from build123d import *

# Parameters (mm, degrees)
SKETCH1_W                                         = 211
SKETCH1_H                                         = 36
BOSS_EXTRUDE1_DEPTH                               = 18
CUT_EXTRUDE1_DEPTH                                = 4
LPATTERN1_COUNT                                   = 9
LPATTERN1_PITCH                                   = 24.4
CBORE_FOR_M2_5_SOCKET_HEAD_CAP_SCREW1_D           = 2.9
CBORE_FOR_M2_5_SOCKET_HEAD_CAP_SCREW1_CBORE_D     = 5.5
CBORE_FOR_M2_5_SOCKET_HEAD_CAP_SCREW1_CBORE_DEPTH = 2.9
FILLET1_R                                         = 2


with BuildPart() as part:
    # Sketch1 → Boss-Extrude1 (new body)
    with BuildSketch(Plane(origin=(0, 0, 0), x_dir=(1, 0, 0), z_dir=(0, 1, 0))):
        Rectangle(SKETCH1_W, SKETCH1_H)
    extrude(amount=BOSS_EXTRUDE1_DEPTH)

    # Sketch2 → Cut-Extrude1 (cut)
    with BuildSketch(Plane(origin=(0, 18, 0), x_dir=(1, 0, 0), z_dir=(0, 1, 0))):
        with BuildLine():
            Line((-101.6, 9.25), (-101.6, -9.25))
            ThreePointArc((-101.6, -9.25), (-97.6, -13.25), (-93.6, -9.25))
            Line((-93.6, -9.25), (-93.6, 9.25))
            ThreePointArc((-93.6, 9.25), (-97.6, 13.25), (-101.6, 9.25))
        make_face()
    cut_extrude1 = extrude(amount=-CUT_EXTRUDE1_DEPTH, mode=Mode.SUBTRACT)

    # LPattern1: Cut-Extrude1 ×9
    with Locations(*[(i * LPATTERN1_PITCH, 0, 0) for i in range(1, LPATTERN1_COUNT)]):
        add(cut_extrude1, mode=Mode.SUBTRACT)

    # CBORE for M2.5 Socket Head Cap Screw1 (through all)
    with Locations(Plane(origin=(0, 18, 0), x_dir=(1, 0, 0), z_dir=(0, 1, 0))):
        with Locations((-85.4, 0), (85.4, 0)):
            CounterBoreHole(CBORE_FOR_M2_5_SOCKET_HEAD_CAP_SCREW1_D / 2, CBORE_FOR_M2_5_SOCKET_HEAD_CAP_SCREW1_CBORE_D / 2, CBORE_FOR_M2_5_SOCKET_HEAD_CAP_SCREW1_CBORE_DEPTH)

    # Fillet1
    fillet1_edges = [part.edges().sort_by_distance(p)[0] for p in [
        (105.5, 9, 18),
        (-105.5, 9, 18),
        (-105.5, 9, -18),
        (105.5, 9, -18),
    ]]
    fillet(fillet1_edges, radius=FILLET1_R)


solid = part.part
The model under review builds one solid part; all positions refer to its coordinate system, in mm. A direction names the side the tool comes from. Give positions to 0.01 mm unless a question says otherwise; leave off trailing zeros. Order: outer loops, then holes, each group sorted by start corner. A loop starts at its lowest first (then second) coordinate and runs counter-clockwise, first axis right, second up. Notation, with made-up numbers: M -39,9 L 7,9 A30 ccw 7,45 Z; hole C -33.75,48.5 d6. An arc over 180 degrees is marked long. Use one line per item in the form item = value. Start each with the question number.
Item 1: For faces 1 (the flat face through (-1, 9, 18)), 2 (the flat face through (-49, 14, 0)), list the 3-axis set-ups (+Z, -Z, +X, -X, +Y, -Y) from which the entire face can be reached by the end or side of a thin tool; tool diameter is ignored.
Item 2: We need section A-A on x = -73.2. Give the boundary of the cut face in (y, z).
Item 3: Insertion check: pin 1 Ø2.5 at (x, z) = (-25, -6) entering from +Y; pin 2 Ø3 at (x, z) = (86, -1) entering from +Y. Each pin has a flat end and moves straight along its axis. Give the tip position at first contact, or say it passes through.
Item 4: The part is to be moulded in two halves that separate along X. For faces 3 (the cylindrical face through (97.69, 16.03, -13.25)), 4 (the flat face through (105.5, 9, 0)), 5 (the flat face through (-1, 0, 0)), 6 (the flat face through (98, 14, 0)), say which applies: pulls with the +X half, pulls with the -X half, needs draft (parallel to the pull), parting line crosses it, or undercut.
Item 5: To check wall thickness, follow line 1 along Z through (x, y) = (-85.4, 12.25); line 2 along Z through (x, y) = (-85.4, 16.25); line 3 along Y through (x, z) = (75, 1.5). State the ranges of each line that lie inside material, in increasing order. Write a range as from..to.
Item 6: We need section B-B on x = 50. Give the boundary of the cut face in (y, z), plus the area to 3 significant figures.
Completed:
q1.face_1 = +Z, +X, -X, +Y, -Y
q1.face_2 = +Y
q2.outline = M 0,-18 L 18,-18 L 18,-13.25 L 14,-13.25 L 14,13.25 L 18,13.25 L 18,18 L 0,18 Z
q3.pin_1 = 14
q3.pin_2 = 15.1
q4.face_3 = undercut
q4.face_4 = pulls with the +X half
q4.face_5 = needs draft
q4.face_6 = undercut
q5.line_1 = -18..-1.45, 1.45..18
q5.line_2 = -18..-2.75, 2.75..18
q5.line_3 = 0..14
q6.outline = M 0,-18 L 18,-18 L 18,-13.07 L 14,-13.07 L 14,13.07 L 18,13.07 L 18,18 L 0,18 Z
q6.area = 543 mm²
